from build123d import *

# Parameters (mm, degrees)
FILLET1_R    = 0.2
SKETCH3_W    = 1.03
SKETCH3_H    = 4.3
SKETCH4_W    = 1.03
SKETCH4_H    = 1.966638464
RECPAT_COUNT = 2
RECPAT_ANGLE = 90


with BuildPart() as part:
    # BodySke → Base-Revolve (revolve)
    with BuildSketch(Plane.XY):
        with BuildLine():
            Line((3.1, 2), (3.1, 4))
            Line((3.1, 4), (1.555305874, 4))
            ThreePointArc((1.555305874, 4), (1.392873227, 3.961271902), (1.265388955, 3.853420195))
            ThreePointArc((1.265388955, 3.853420195), (0.324444487, 2.027933456), (0, 0))
            Line((0, 0), (58.1, 0))
            Line((58.1, 0), (58.1, 2))
            Line((58.1, 2), (3.1, 2))
        make_face()
    revolve(axis=Axis((-25.4, 0, 0), (1, 0, 0)))

    # Fillet1
    fillet1_edges = [part.edges().sort_by_distance(p)[0] for p in [
        (3.1, -2, 0),
    ]]
    fillet(fillet1_edges, radius=FILLET1_R)

    # Sketch3 → Recess section 0
    with BuildSketch(Plane(origin=(0, 0, 0), x_dir=(0, 0, -1), z_dir=(1, 0, 0))):
        Rectangle(SKETCH3_W, SKETCH3_H)
    # Sketch4 → Recess section 1
    with BuildSketch(Plane(origin=(2.34, 0, 0), x_dir=(0, 0, -1), z_dir=(1, 0, 0))):
        Rectangle(SKETCH4_W, SKETCH4_H)
    recess = loft(mode=Mode.SUBTRACT)

    # RecPat: Recess ×2 about axis
    recpat_axis = Axis((0, 0, 0), (1, 0, 0))
    for i in range(1, RECPAT_COUNT):
        add(recess.rotate(recpat_axis, i * RECPAT_ANGLE / (RECPAT_COUNT - 1)), mode=Mode.SUBTRACT)

    # RecCorSke → RecessCore (revolve, cut)
    with BuildSketch(Plane.XY):
        Polygon((0, 0), (0, 1.01462874), (2.34, 0.851), (2.616506661, 0), align=None)
    revolve(axis=Axis((-3.175, 0, 0), (1, 0, 0)), mode=Mode.SUBTRACT)


solid = part.part
For this review, take the finished solid that the model builds, in its own axes (mm). A direction names the side the tool comes from. Round coordinates to 2 decimals unless told otherwise and drop trailing zeros. Order: outer loops, then holes, each group sorted by start corner. A loop starts at its lowest first (then second) coordinate and runs counter-clockwise, first axis right, second up. Notation, with made-up numbers: (39.25, 58) -> (81.25, 58) arc R14 cw to (81.25, 71) -> close; hole circle Ø9 at (-38, -22). An arc over 180 degrees is marked (long way). Write item = value, one per line. Start each with the question number.
1) Take a section at A-A on x = 35.5. State the section outline as (y, z) points.
2) Insertion check: pin 1 (4 mm diameter, centred on x = 14.5, y = -2.5, fed in from -Z); pin 2 (1 mm diameter, centred on x = 13.5, y = 0.5, fed in from -Z); pin 3 (3 mm diameter, centred on x = 36.5, z = -1.5, fed in from +Y). Each pin has a flat end and moves straight along its axis. Give the tip position at first contact, or say it passes through.
3) Tool access review of faces 4 (the face through (58.1, 0, 0)), 5 (the face through (1.3, -1.5, 0)): name each direction out of +Z, -Z, +X, -X, +Y, -Y from which nothing blocks a thin tool from reaching the whole face with its end or side.
4) The part is to be moulded in two halves that separate along Y. For faces 1 (the face through (2.6, 0.04, -0.02)), 2 (the face through (30, 0, -2)), 3 (the face through (3.1, -2, -2)), say which applies: +Y half, -Y half, draft (parallel to the pull), parting line (faces both ways), or undercut.
5) To check wall thickness, follow line 1 (X direction, y = -0.5, z = -2.5); line 2 (X direction, y = -1.25, z = 0.25); line 3 (Y direction, x = 5.5, z = -0.5). State the ranges of each line that lie inside material, in increasing order. Write a range as from..to.
Verdict:
q1.outline = circle Ø4 at (0, 0)
q2.pin_1 = -1.94
q2.pin_2 = -2
q2.pin_3 = 2
q3.face_4 = +Z, -Z, +X, +Y, -Y
q3.face_5 = -X
q4.face_1 = undercut
q4.face_2 = parting line
q4.face_3 = draft
q5.line_1 = 0.52..3.1
q5.line_2 = 1.81..58.1
q5.line_3 = -1.94..1.94
